Work out the finished part from the listing and answer in its coordinate system (mm). A direction names the side the tool comes from. Give positions to 0.01 mm unless a question says otherwise; leave off trailing zeros. Write each loop counter-clockwise with the first axis right and the second up, starting at its lowest first coordinate (ties: lowest second). Pieces come first, ordered by that corner, then holes.
1) Find section A-A (z = -35). Determine the outline of the cut face in (x, y).
2) Find section D-D (y = 5). Determine the outline of the cut face in (x, z), plus the area to 3 significant figures.
3) Find section C-C (x = 14.5). Determine the outline of the cut face in (y, z).
4) Given pin 1 Ø3 at (y, z) = (15.5, -34.5) entering from +X; pin 2 Ø3.5 at (x, y) = (15.07, 9) entering from +Z; pin 3 Ø4 at (x, y) = (15.5, 11.5) entering from -Z; pin 4 Ø1.5 at (x, z) = (18.5, -32.5) entering from +Y, each flat-ended and moving along its own axis, determine where each tip first touches the part or whether it passes through.
5) Determine the mould class of faces 5 (the face through (13, 7, -30.128)), 6 (the face through (15, 0.6, -28.7)), 7 (the face through (17.069, 2, -34)) for opening direction Y: pulls with the +Y half, pulls with the -Y half, needs draft (parallel to the pull), parting line crosses it, or undercut.
6) Straight lines are drawn through the part: probe 1 along Y at (x, z) = (13.5, -31.75); probe 2 along Y at (x, z) = (16, -34.25); probe 3 along Z at (x, y) = (12.75, 15.75). For each, find the intervals that lie inside material, in ascending order.
7) A tool of negligible diameter and unlimited length cuts with its end or side. For faces 1 (the face through (10.569, 16, -36)), 2 (the face through (19.866, 1.141, -31.607)), 3 (the face through (13.069, 16, -34)), 4 (the face through (18.11, 7.27, -31.65)), from which of +Z, -Z, +X, -X, +Y, -Y can it reach the whole face along a straight path? Write none if from no direction.
8) Find section B-B (z = -30.75). Determine the outline of the cut face in (x, y), plus the area to 3 significant figures.
```python
from build123d import *

# Parameters (mm, degrees)
BOSS_EXTRU_3_DEPTH      = 4
ESQUISSE3_W             = 12
ESQUISSE3_H             = 5
BOSS_EXTRU_4_DEPTH      = 5
ENL_V_MAT_EXTRU_1_REACH = 7
ESQUISSE4_R             = 2.2
ENL_V_MAT_EXTRU_2_DEPTH = 3
CONG_1_R                = 4
CONG_2_R                = 2


with BuildPart() as part:
    # Esquisse2 → Boss.-Extru.3 (new body)
    with BuildSketch(Plane(origin=(0, 0, 0), x_dir=(1, 0, 0), z_dir=(0, 1, 0))):
        with BuildLine():
            Line((11.568725398, 38.128215269), (18.568725398, 38.128215269))
            ThreePointArc((18.568725398, 38.128215269), (19.275832179, 37.83532205), (19.568725398, 37.128215269))
            Line((19.568725398, 37.128215269), (19.568725398, 35.628215269))
            Line((19.568725398, 35.628215269), (17.068725398, 35.628215269))
            Line((17.068725398, 35.628215269), (17.068725398, 33.128215269))
            Line((17.068725398, 33.128215269), (21.068725398, 33.128215269))
            Line((21.068725398, 33.128215269), (21.068725398, 28.128215269))
            Line((21.068725398, 28.128215269), (9.068725398, 28.128215269))
            Line((9.068725398, 28.128215269), (9.068725398, 33.128215269))
            Line((9.068725398, 33.128215269), (13.068725398, 33.128215269))
            Line((13.068725398, 33.128215269), (13.068725398, 35.628215269))
            Line((13.068725398, 35.628215269), (10.568725398, 35.628215269))
            Line((10.568725398, 35.628215269), (10.568725398, 37.128215269))
            ThreePointArc((10.568725398, 37.128215269), (10.861618616, 37.83532205), (11.568725398, 38.128215269))
        make_face()
    extrude(amount=BOSS_EXTRU_3_DEPTH)

    # Esquisse3 → Boss.-Extru.4 (add)
    with BuildSketch(Plane(origin=(0, 4, 0), x_dir=(1, 0, 0), z_dir=(0, 1, 0))):
        with Locations((15.068725398, 30.628215269)):
            Rectangle(ESQUISSE3_W, ESQUISSE3_H)
    extrude(amount=BOSS_EXTRU_4_DEPTH)

    # Symétrie1: part across plane


with BuildPart() as part_1:
    add(part.part)
    add(part.part.mirror(Plane.ZX.offset(9)))

    # Esquisse4 → Enlèv. mat.-Extru.1 (cut, up to next)
    with BuildSketch(Plane(origin=(0, 0, -33.128215269), x_dir=(-1, 0, 0), z_dir=(0, 0, -1)), mode=Mode.PRIVATE) as enl_v_mat_extru_1_sk1:
        with Locations((-15.068725398, 9)):
            Circle(ESQUISSE4_R)
    enl_v_mat_extru_1_tool1 = extrude(enl_v_mat_extru_1_sk1.sketch, amount=-ENL_V_MAT_EXTRU_1_REACH, mode=Mode.PRIVATE) & part_1.part
    add(enl_v_mat_extru_1_tool1.solids().sort_by_distance((15.068725, 9, -33.128215))[0], mode=Mode.SUBTRACT)

    # Esquisse5 → Enlèv. mat.-Extru.2 (cut)
    with BuildSketch(Plane(origin=(0, 0, -33.128215269), x_dir=(-1, 0, 0), z_dir=(0, 0, -1))):
        Polygon((-13.047999455, 12.5), (-17.08945134, 12.5), (-19.110177282, 9), (-17.08945134, 5.5), (-13.047999455, 5.5), (-11.027273513, 9), align=None)
    extrude(amount=-ENL_V_MAT_EXTRU_2_DEPTH, mode=Mode.SUBTRACT)

    # Congé1
    cong_1_edges = [part_1.edges().sort_by_distance(p)[0] for p in [
        (9.068725398, 0, -30.628215269),
        (9.068725398, 18, -30.628215269),
        (21.068725398, 18, -30.628215269),
        (21.068725398, 0, -30.628215269),
    ]]
    fillet(cong_1_edges, radius=CONG_1_R)

    # Congé2
    cong_2_edges = [part_1.edges().sort_by_distance(p)[0] for p in [
        (9.068725398, 9, -28.128215269),
        (15.068725398, 0, -28.128215269),
        (21.068725398, 9, -28.128215269),
        (15.068725398, 18, -28.128215269),
        (19.897152522, 16.828427125, -28.128215269),
        (19.897152522, 1.171572875, -28.128215269),
        (10.240298273, 16.828427125, -28.128215269),
        (10.240298273, 1.171572875, -28.128215269),
    ]]
    fillet(cong_2_edges, radius=CONG_2_R)


solid = part_1.part
```
Results:
1. outline: (13.07, 0) - (17.07, 0) - (17.07, 4) - (13.07, 4) - close; (13.07, 14) - (17.07, 14) - (17.07, 18) - (13.07, 18) - close
2. outline: (9.07, -33.13) - (21.07, -33.13) - (21.07, -30.13) arc R2 ccw to (19.07, -28.13) - (11.07, -28.13) arc R2 ccw to (9.07, -30.13) - close
2. area: 58.3 mm2
3. outline: (0, -38.13) - (4, -38.13) - (4, -33.13) - (5.5, -33.13) - (5.5, -30.13) - (6.87, -30.13) - (6.87, -28.13) - (2, -28.13) arc R2 ccw to (0, -30.13) - close; (11.13, -30.13) - (12.5, -30.13) - (12.5, -33.13) - (14, -33.13) - (14, -38.13) - (18, -38.13) - (18, -30.13) arc R2 ccw to (16, -28.13) - (11.13, -28.13) - close
4. pin 1: stops at x = 20.97
4. pin 2: passes through
4. pin 3: stops at z = -33.13
4. pin 4: stops at y = 17.94
5. face 5: undercut
5. face 6: pulls with the -Y half
5. face 7: needs draft
6. probe 1: y = 0 to 5.5, 12.5 to 18
6. probe 2: y = 0 to 4, 14 to 18
6. probe 3: z = -38.13 to -35.63, -33.13 to -28.13
7. face 1: -Z, -X, +Y, -Y
7. face 2: +Z, +X, -Y
7. face 3: -X, +Y, -Y
7. face 4: -Z
8. outline: (9.07, 4) arc R4 ccw to (13.07, 0) - (17.07, 0) arc R4 ccw to (21.07, 4) - (21.07, 14) arc R4 ccw to (17.07, 18) - (13.07, 18) arc R4 ccw to (9.07, 14) - close; hole (11.03, 9) - (13.05, 5.5) - (17.09, 5.5) - (19.11, 9) - (17.09, 12.5) - (13.05, 12.5) - close
8. area: 160 mm2
